Read the model definition and answer for the solid it produces. Units are mm, in the model's axes. Coordinates: 2 decimals unless noted, no trailing zeros. Write each loop counter-clockwise with the first axis right and the second up, starting at its lowest first coordinate (ties: lowest second). Pieces come first, ordered by that corner, then holes. Notation, with made-up numbers: (58, 14.25) -> (94, 14.25) arc R8 ccw to (94, 27.25) -> close; hole circle Ø1 at (35, -34.75). An arc over 180 degrees is marked (long way). One line per item, written item: value. Start each with the question number.
1. Given P1, Ø1.5, axis at y = 17, z = 2, coming from the -X side, flat-ended and moving along its own axis, determine where the tip first touches the part or whether it passes through.
2. For a pull along Y with two mould halves and no side action, classify faces 1 (the cylindrical face through (8.89, 18.01, 2.54)), 2 (the flat face through (120, 10, 2)), 3 (the flat face through (64, 0, 2)), 4 (the cylindrical face through (15.5, 10.07, 2.54)) as pulls with the +Y half, pulls with the -Y half, needs draft (parallel to the pull), parting line crosses it, or undercut.
3. Find section A-A, the plane x = 17. Write down the section's boundary in (y, z), and give its area (3 significant figures).
4. Find section D-D, the plane x = 3. Write down the section's boundary in (y, z), and give its area (3 significant figures).
5. Find section C-C, the plane z = 2.3. Write down the section's boundary in (x, y) (3 decimals).
6. Consider line 1 along Y through (x, z) = (10, 1.3) (3 decimals); line 2 along Y through (x, z) = (17, 2.5); line 3 along X through (y, z) = (10.25, 1.95). Determine where each line is inside the solid, lowest interval first.
7. Find section B-B, the plane y = 10. Write down the section's boundary in (x, z) (3 decimals), and give its area (3 significant figures).
```python
from build123d import *

# Parameters (mm, degrees)
SKETCH1_W           = 120
SKETCH1_H           = 20
BOSS_EXTRUDE1_DEPTH = 5
SKETCH2_R           = 1.5
SKETCH2_R_2         = 3.025
CUT_EXTRUDE1_DEPTH  = 10
CUT_EXTRUDE2_DEPTH  = 10
SKETCH5_R           = 2
CUT_EXTRUDE3_DEPTH  = 10


with BuildPart() as part:
    # Sketch1 → Boss-Extrude1 (new body)
    with BuildSketch(Plane.XY):
        with Locations((60, 10)):
            Rectangle(SKETCH1_W, SKETCH1_H)
    extrude(amount=BOSS_EXTRUDE1_DEPTH)

    # Sketch2 → Cut-Extrude1 (cut)
    with BuildSketch(Plane.XY.offset(5)):
        with Locations((10, 17)):
            Circle(SKETCH2_R)
        with Locations((17, 10)):
            Circle(SKETCH2_R)
        with Locations((10, 10)):
            Circle(SKETCH2_R_2)
        with Locations((10, 3)):
            Circle(SKETCH2_R)
        with Locations((3, 10)):
            Circle(SKETCH2_R)
    extrude(amount=-CUT_EXTRUDE1_DEPTH, mode=Mode.SUBTRACT)

    # Sketch3 → Cut-Extrude2 (cut)
    with BuildSketch(Plane.XY.offset(5)):
        with BuildLine():
            Line((10, 30), (10, 20))
            ThreePointArc((10, 20), (0, 10), (10, 0))
            Line((10, 0), (10, -10))
            ThreePointArc((10, -10), (-10, 10), (10, 30))
        make_face()
    extrude(amount=-CUT_EXTRUDE2_DEPTH, mode=Mode.SUBTRACT)

    # Sketch5 → Cut-Extrude3 (cut)
    with BuildSketch(Plane.XY.offset(5)):
        with Locations((115, 15)):
            Circle(SKETCH5_R)
        with Locations((115, 5)):
            Circle(SKETCH5_R)
    extrude(amount=-CUT_EXTRUDE3_DEPTH, mode=Mode.SUBTRACT)


solid = part.part
```
Answer block:
1. P1: stops at x = 2.19
2. face 1: undercut
2. face 2: needs draft
2. face 3: pulls with the -Y half
2. face 4: undercut
3. outline: (0, 0) -> (8.5, 0) -> (8.5, 5) -> (0, 5) -> close; (11.5, 0) -> (20, 0) -> (20, 5) -> (11.5, 5) -> close
3. area: 85.0 mm2
4. outline: (2.86, 0) -> (8.5, 0) -> (8.5, 5) -> (2.86, 5) -> close; (11.5, 0) -> (17.14, 0) -> (17.14, 5) -> (11.5, 5) -> close
4. area: 56.4 mm2
5. outline: (10, 0) -> (120, 0) -> (120, 20) -> (10, 20) arc R10 ccw to start; hole circle Ø3 at (3, 10); hole circle Ø6.05 at (10, 10); hole circle Ø3 at (10, 3); hole circle Ø3 at (10, 17); hole circle Ø3 at (17, 10); hole circle Ø4 at (115, 5); hole circle Ø4 at (115, 15)
6. line 1: y = 0 to 1.5, 4.5 to 6.975, 13.025 to 15.5, 18.5 to 20
6. line 2: y = 0 to 8.5, 11.5 to 20
6. line 3: x = 0 to 1.52, 4.48 to 6.99, 13.01 to 15.52, 18.48 to 120
7. outline: (0, 0) -> (1.5, 0) -> (1.5, 5) -> (0, 5) -> close; (4.5, 0) -> (6.975, 0) -> (6.975, 5) -> (4.5, 5) -> close; (13.025, 0) -> (15.5, 0) -> (15.5, 5) -> (13.025, 5) -> close; (18.5, 0) -> (120, 0) -> (120, 5) -> (18.5, 5) -> close
7. area: 540 mm2
